```python
from build123d import *

# Parameters (mm, degrees)
F1_DEPTH  = 1.45
F2_R      = 8.05
F2_R_2    = 5
F3_DEPTH  = 5
F4_W      = 3.1
F4_H      = 2.9
F6_ANGLE  = -90
F11_R     = 1.45
F12_DEPTH = 25
F14_R     = 1.45
F15_DEPTH = 12.5


with BuildPart() as f1:
    # F0 (on Top) → F1 (new body, symmetric)
    with BuildSketch(Plane.XY):
        with BuildLine():
            ThreePointArc((-3.925, 7.028291), (0, 8.05), (3.925, 7.028291))
            Line((3.925, 7.028291), (3.925, 15.5))
            ThreePointArc((3.925, 15.5), (0, 19.425), (-3.925, 15.5))
            Line((-3.925, 15.5), (-3.925, 7.028291))
        make_face()
    extrude(amount=F1_DEPTH, both=True)

    # F2 (on Top) → F3 (join, symmetric)
    with BuildSketch(Plane.XY):
        Circle(F2_R)
        Circle(F2_R_2, mode=Mode.SUBTRACT)
    extrude(amount=F3_DEPTH, both=True)

    # F4 (on Front) → F6 (revolve, symmetric, cut)
    with BuildSketch(Plane.XZ) as f6_sk:
        with Locations((-6.5, 0)):
            Rectangle(F4_W, F4_H)
        with Locations((6.5, 0)):
            Rectangle(F4_W, F4_H)
    revolve(axis=Axis((0, 0, 0.165465), (0, 0, 1)), revolution_arc=F6_ANGLE / 2, mode=Mode.SUBTRACT)
    revolve(f6_sk.sketch, axis=Axis((0, 0, 0.165465), (0, 0, -1)), revolution_arc=F6_ANGLE / 2, mode=Mode.SUBTRACT)

    # F7 (on Right) → F8 (revolve)
    with BuildSketch(Plane.YZ):
        with BuildLine():
            Line((14, 1.45), (15.5, 1.45))
            Line((15.5, 1.45), (15.5, 6.5))
            Line((15.5, 6.5), (15.5, 8.425))
            ThreePointArc((15.5, 8.425), (13.701718, 7.186883), (14.216667, 5.06519))
            Line((14.216667, 5.06519), (14, 1.45))
        make_face()
    revolve(axis=Axis((0, 15.5, 3.25), (0, 0, 1)))

    # F11 (on face) → F12 (cut)
    with BuildSketch(Plane(origin=(7.946074, 7.946074, 0), x_dir=(-0.707107, 0.707107, 0), z_dir=(0.707107, 0.707107, 0))):
        Circle(F11_R)
    extrude(amount=-F12_DEPTH, mode=Mode.SUBTRACT)

    # F14 (on face) → F15 (cut, symmetric)
    with BuildSketch(Plane(origin=(0, 0, 0), x_dir=(0.707107, 0.707107, 0), z_dir=(0.707107, -0.707107, 0))):
        Circle(F14_R)
    extrude(amount=F15_DEPTH, both=True, mode=Mode.SUBTRACT)


solid = f1.part
```
The listing builds one solid part. Answer for the finished solid, in the listing's coordinates (mm). A direction names the side the tool comes from. Give positions to 0.01 mm unless a question says otherwise; leave off trailing zeros. Write each loop counter-clockwise with the first axis right and the second up, starting at its lowest first coordinate (ties: lowest second). Pieces come first, ordered by that corner, then holes. Notation, with made-up numbers: M 84.5,49.25 L 128.5,49.25 A12 ccw 128.5,71.25 Z; hole C -21.75,89 d4. An arc over 180 degrees is marked long. Write each question's results on one line, items separated by ' | '.
Q1. Section C-C, the plane x = 6 is taken. Write down the section's boundary in (y, z).
Output values:
outline: M -5.37,-5 L 5.37,-5 L 5.37,-1.45 L -5.37,-1.45 Z; M -5.37,1.45 L 5.37,1.45 L 5.37,5 L -5.37,5 Z
Q2. Consider L1, parallel to Y at x = 0, z = 1.5; L2, parallel to Y at x = 0, z = -1 (3 decimals); L3, parallel to X at y = 0, z = -1.5. Determine where each line is inside the solid, lowest interval first. Write a range as from..to.
Output values:
L1: -8.05..-5, 5..8.05, 14..17 | L2: -8.05..-5, 5..19.425 | L3: -8.05..-5, 5..8.05
Q3. Section D-D, the plane z = 4.25 is taken. Write down the section's boundary in (x, y), then the cut area to 3 significant figures.
Output values:
outline: C 0,0 d16.1; C 0,15.5 d2.66; hole C 0,0 d10 | area: 131 mm2
Q4. A tool of negligible diameter and unlimited length cuts with its end or side. For faces 1 (the flat face through (-3.925, 11, 0)), 2 (the flat face through (6, 0, 1.45)), 3 (the conical face through (-0.53, 14.21, 3.23)), 4 (the cylindrical face through (-3.5, 5.55, -0.03)), from which of +Z, -Z, +X, -X, +Y, -Y can it reach the whole face along a straight path? Write none if from no direction.
Output values:
face 1: +Z, -Z, -X, +Y | face 2: +X | face 3: none | face 4: -X
Q5. Section A-A, the plane y = 0 is taken. Write down the section's boundary in (x, z).
Output values:
outline: M -8.05,-5 L -5,-5 L -5,-1.45 L -8.05,-1.45 Z; M -8.05,1.45 L -5,1.45 L -5,5 L -8.05,5 Z; M 5,-5 L 8.05,-5 L 8.05,-1.45 L 5,-1.45 Z; M 5,1.45 L 8.05,1.45 L 8.05,5 L 5,5 Z
Q6. For a pull along Z with two mould halves and no side action, classify faces 5 (the flat face through (3.925, 11, 0)), 6 (the flat face through (-0.1, -5.3, 5)), 7 (the cylindrical face through (-3.49, -5.54, 0.03)) as released by +Z, released by -Z, zero draft, split by the parting line, or undercut.
Output values:
face 5: zero draft | face 6: released by +Z | face 7: undercut
Q7. Flat-ended cylindrical pins translate along their axes: P1, Ø6, axis at y = 1.5, z = 0, coming from the +X side; P2, Ø5, axis at x = -5.5, y = 1.5, coming from the +Z side; P3, Ø1.4, axis at y = 11, z = 0, coming from the +X side (3 decimals); P4, Ø2, axis at y = 7, z = 0.5, coming from the +X side. Find the tip coordinate at first contact, or state that the pin passes through.
Output values:
P1: x = 8.05 | P2: z = 5 | P3: x = 3.925 | P4: x = 5.06
Q8. Section B-B, the plane z = 0.5 is taken. Write down the section's boundary in (x, y) (3 decimals).
Output values:
outline: M -4.648,-6.573 A8.05 ccw 4.648,-6.573 L 2.44,-4.364 A5 cw -2.44,-4.364 Z; M -4.648,6.573 L -2.44,4.364 A5 cw 2.44,4.364 L 4.648,6.573 A8.05 ccw 3.925,7.028 L 3.925,15.5 A3.925 ccw -3.925,15.5 L -3.925,7.028 A8.05 ccw Z
